from build123d import *

# Parameters (mm, degrees)
SKETCH1_R           = 6
BOSS_EXTRUDE1_DEPTH = 100
CUT_EXTRUDE1_DEPTH  = 101
FILLET1_R           = 1


with BuildPart() as part:
    # Sketch1 → Boss-Extrude1 (new body)
    with BuildSketch(Plane(origin=(0, 0, 0), x_dir=(0, 0, -1), z_dir=(1, 0, 0))):
        Circle(SKETCH1_R)
    extrude(amount=BOSS_EXTRUDE1_DEPTH)

    # Sketch2 → Cut-Extrude1 (cut, through all)
    with BuildSketch(Plane(origin=(100, 0, 0), x_dir=(0, 0, -1), z_dir=(1, 0, 0))):
        Polygon((45.463107393, 6.099427515), (3.968626967, 6.099427515), (-3.968626967, 6.099427515), (-3.968626967, 4.5), (3.968626967, 4.5), (3.968626967, 6.19024408), (3.968626967, 47.684724507), (-54.777541729, -10.933150643), (-13.283061303, -52.518447634), align=None)
    extrude(amount=-CUT_EXTRUDE1_DEPTH, mode=Mode.SUBTRACT)

    # Fillet1
    fillet1_edges = [part.edges().sort_by_distance(p)[0] for p in [
        (50, 4.5, 3.968626967),
        (50, 4.5, -3.968626967),
    ]]
    fillet(fillet1_edges, radius=FILLET1_R)


solid = part.part
Source: CAD feature listing. Evaluate the final solid. Frame: model axes, mm. Round coordinates to 2 decimals unless told otherwise and drop trailing zeros. Loops run counter-clockwise (first coordinate to the right, second up) from the corner with the lowest first, then second, coordinate; pieces in that order, holes last. Notation, with made-up numbers: (-20.5, 72.25) - (30.5, 72.25) arc R12 cw to (30.5, 81.25) - close; hole circle Ø2 at (-17.75, 41.5). An arc over 180 degrees is marked (long way). Write item = value, one per line. Start each with the question number.
(1) Pull-direction query (X, two-part tool) for faces 1 (the face through (49, -6, 0)), 2 (the face through (0, -1, 0)), 3 (the face through (100, -1, 0)); classes: +X half, -X half, draft (parallel to the pull), parting line (faces both ways), or undercut.
(2) Pin query (flat end, axial travel): pin 1 (3 mm diameter, centred on x = 14, z = 1.5, fed in from -Y); pin 2 (2 mm diameter, centred on x = 73, y = -2, fed in from +Z). Return the tip coordinate at first contact, or that it passes through.
(3) Section query A-A, the plane y = 1.75. Output: boundary loops of the cut face in (x, z), plus the area to 3 significant figures.
(4) Ray query, line 1 along Z through (x, y) = (85.5, 0.25); line 2 along Z through (x, y) = (67.5, -1.5); line 3 along Y through (x, z) = (18.5, -2). Return the intervals inside material, ascending. Write a range as from..to.
(5) Section query B-B, the plane x = 14.5. Output: boundary loops of the cut face in (y, z), plus the area to 3 significant figures.
Conclusion:
q1.face_1 = draft
q1.face_2 = -X half
q1.face_3 = +X half
q2.pin_1 = -6
q2.pin_2 = 5.92
q3.outline = (0, -5.74) - (100, -5.74) - (100, 5.74) - (0, 5.74) - close
q3.area = 1,150 mm2
q4.line_1 = -5.99..5.99
q4.line_2 = -5.81..5.81
q4.line_3 = -5.66..4.5
q5.outline = (4.2, -4.28) arc R1 ccw to (4.5, -3.57) - (4.5, 3.57) arc R1 ccw to (4.2, 4.28) arc R6 ccw (long way) to start
q5.area = 105 mm2
